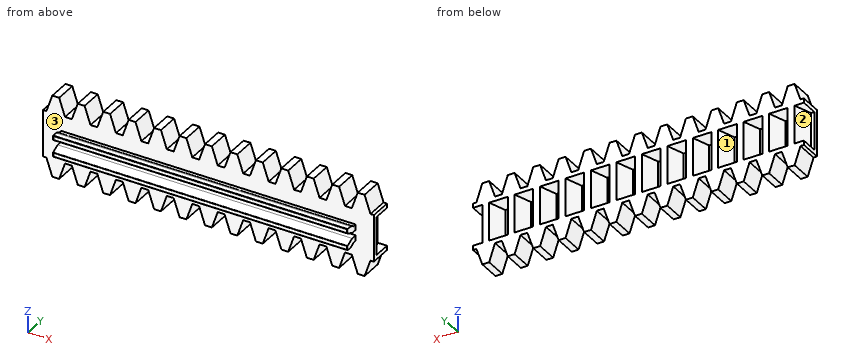
```python
from build123d import *

# Parameters (mm, degrees)
SKETCH_1_W                     = 4.65
SKETCH_1_H                     = 8.6
EXTRUDE_1_DEPTH                = 4
EXTRUDE_2_DEPTH                = 4
CUT_EXTRUDE_1_DEPTH            = 3.5
PATTERN_LINEAR_4_COUNT         = 13
PATTERN_LINEAR_4_PITCH         = 4.65
PATTERN_LINEAR_4_COPY_1_DEPTH  = 4
PATTERN_LINEAR_4_COPY_2_DEPTH  = 4
PATTERN_LINEAR_4_COPY_3_DEPTH  = 4
PATTERN_LINEAR_4_COPY_4_DEPTH  = 4
PATTERN_LINEAR_4_COPY_5_DEPTH  = 4
PATTERN_LINEAR_4_COPY_6_DEPTH  = 4
PATTERN_LINEAR_4_COPY_7_DEPTH  = 4
PATTERN_LINEAR_4_COPY_8_DEPTH  = 4
PATTERN_LINEAR_4_COPY_9_DEPTH  = 4
PATTERN_LINEAR_4_COPY_10_DEPTH = 4
PATTERN_LINEAR_4_COPY_11_DEPTH = 4
PATTERN_LINEAR_4_COPY_12_DEPTH = 4
EXTRUDE_START                  = 1
EXTRUDE_4_DEPTH                = 53.8
FILLET_1_R                     = 0.1


with BuildPart() as part:
    # 草图1 → 凸台-拉伸1 (new body)
    with BuildSketch(Plane(origin=(0, 0, 0), x_dir=(1, 0, 0), z_dir=(0, 1, 0))):
        Rectangle(SKETCH_1_W, SKETCH_1_H)
    extrude_1 = extrude(amount=EXTRUDE_1_DEPTH)

    # 草图3 → 凸台-拉伸2 (add)
    with BuildSketch(Plane(origin=(0, 0, 0), x_dir=(1, 0, 0), z_dir=(0, 1, 0))):
        Polygon((0.625, 7.5), (-0.625, 7.5), (-1.7, 4.3), (1.7, 4.3), align=None)
    extrude_2 = extrude(amount=EXTRUDE_2_DEPTH)

    # 镜向1: 凸台-拉伸2 across plane
    add(extrude_2.mirror(Plane.XY))

    # 草图4 → 切除-拉伸1 (cut, symmetric)
    with BuildSketch(Plane.XY):
        Polygon((-0.625, 4), (-2.325, 4), (-2.325, 0.8), (-1.7, 0.8), align=None)
        Polygon((1.7, 0.8), (2.325, 0.8), (2.325, 4), (0.625, 4), align=None)
    cut_extrude_1 = extrude(amount=CUT_EXTRUDE_1_DEPTH, both=True, mode=Mode.SUBTRACT)

    # 阵列(线性)4: 凸台-拉伸1, 凸台-拉伸2, 切除-拉伸1 ×13
    with Locations(*[(i * PATTERN_LINEAR_4_PITCH, 0, 0) for i in range(1, PATTERN_LINEAR_4_COUNT)]):
        add(extrude_1)
        add(extrude_2)
        add(cut_extrude_1, mode=Mode.SUBTRACT)

    # 阵列(线性)4 copy 1 sketch → 阵列(线性)4 copy 1 (add)
    with BuildSketch(Plane(origin=(4.65, 0, 0), x_dir=(1, 0, 0), z_dir=(0, 1, 0))):
        Polygon((0.625, -7.5), (-0.625, -7.5), (-1.7, -4.3), (1.7, -4.3), align=None)
    extrude(amount=PATTERN_LINEAR_4_COPY_1_DEPTH)

    # 阵列(线性)4 copy 2 sketch → 阵列(线性)4 copy 2 (add)
    with BuildSketch(Plane(origin=(9.3, 0, 0), x_dir=(1, 0, 0), z_dir=(0, 1, 0))):
        Polygon((0.625, -7.5), (-0.625, -7.5), (-1.7, -4.3), (1.7, -4.3), align=None)
    extrude(amount=PATTERN_LINEAR_4_COPY_2_DEPTH)

    # 阵列(线性)4 copy 3 sketch → 阵列(线性)4 copy 3 (add)
    with BuildSketch(Plane(origin=(13.95, 0, 0), x_dir=(1, 0, 0), z_dir=(0, 1, 0))):
        Polygon((0.625, -7.5), (-0.625, -7.5), (-1.7, -4.3), (1.7, -4.3), align=None)
    extrude(amount=PATTERN_LINEAR_4_COPY_3_DEPTH)

    # 阵列(线性)4 copy 4 sketch → 阵列(线性)4 copy 4 (add)
    with BuildSketch(Plane(origin=(18.6, 0, 0), x_dir=(1, 0, 0), z_dir=(0, 1, 0))):
        Polygon((0.625, -7.5), (-0.625, -7.5), (-1.7, -4.3), (1.7, -4.3), align=None)
    extrude(amount=PATTERN_LINEAR_4_COPY_4_DEPTH)

    # 阵列(线性)4 copy 5 sketch → 阵列(线性)4 copy 5 (add)
    with BuildSketch(Plane(origin=(23.25, 0, 0), x_dir=(1, 0, 0), z_dir=(0, 1, 0))):
        Polygon((0.625, -7.5), (-0.625, -7.5), (-1.7, -4.3), (1.7, -4.3), align=None)
    extrude(amount=PATTERN_LINEAR_4_COPY_5_DEPTH)

    # 阵列(线性)4 copy 6 sketch → 阵列(线性)4 copy 6 (add)
    with BuildSketch(Plane(origin=(27.9, 0, 0), x_dir=(1, 0, 0), z_dir=(0, 1, 0))):
        Polygon((0.625, -7.5), (-0.625, -7.5), (-1.7, -4.3), (1.7, -4.3), align=None)
    extrude(amount=PATTERN_LINEAR_4_COPY_6_DEPTH)

    # 阵列(线性)4 copy 7 sketch → 阵列(线性)4 copy 7 (add)
    with BuildSketch(Plane(origin=(32.55, 0, 0), x_dir=(1, 0, 0), z_dir=(0, 1, 0))):
        Polygon((0.625, -7.5), (-0.625, -7.5), (-1.7, -4.3), (1.7, -4.3), align=None)
    extrude(amount=PATTERN_LINEAR_4_COPY_7_DEPTH)

    # 阵列(线性)4 copy 8 sketch → 阵列(线性)4 copy 8 (add)
    with BuildSketch(Plane(origin=(37.2, 0, 0), x_dir=(1, 0, 0), z_dir=(0, 1, 0))):
        Polygon((0.625, -7.5), (-0.625, -7.5), (-1.7, -4.3), (1.7, -4.3), align=None)
    extrude(amount=PATTERN_LINEAR_4_COPY_8_DEPTH)

    # 阵列(线性)4 copy 9 sketch → 阵列(线性)4 copy 9 (add)
    with BuildSketch(Plane(origin=(41.85, 0, 0), x_dir=(1, 0, 0), z_dir=(0, 1, 0))):
        Polygon((0.625, -7.5), (-0.625, -7.5), (-1.7, -4.3), (1.7, -4.3), align=None)
    extrude(amount=PATTERN_LINEAR_4_COPY_9_DEPTH)

    # 阵列(线性)4 copy 10 sketch → 阵列(线性)4 copy 10 (add)
    with BuildSketch(Plane(origin=(46.5, 0, 0), x_dir=(1, 0, 0), z_dir=(0, 1, 0))):
        Polygon((0.625, -7.5), (-0.625, -7.5), (-1.7, -4.3), (1.7, -4.3), align=None)
    extrude(amount=PATTERN_LINEAR_4_COPY_10_DEPTH)

    # 阵列(线性)4 copy 11 sketch → 阵列(线性)4 copy 11 (add)
    with BuildSketch(Plane(origin=(51.15, 0, 0), x_dir=(1, 0, 0), z_dir=(0, 1, 0))):
        Polygon((0.625, -7.5), (-0.625, -7.5), (-1.7, -4.3), (1.7, -4.3), align=None)
    extrude(amount=PATTERN_LINEAR_4_COPY_11_DEPTH)

    # 阵列(线性)4 copy 12 sketch → 阵列(线性)4 copy 12 (add)
    with BuildSketch(Plane(origin=(55.8, 0, 0), x_dir=(1, 0, 0), z_dir=(0, 1, 0))):
        Polygon((0.625, -7.5), (-0.625, -7.5), (-1.7, -4.3), (1.7, -4.3), align=None)
    extrude(amount=PATTERN_LINEAR_4_COPY_12_DEPTH)

    # 草图6 → 凸台-拉伸4 (add)
    with BuildSketch(Plane(origin=(0, 0, 0), x_dir=(0, 0, -1), z_dir=(1, 0, 0)).offset(EXTRUDE_START)):
        with BuildLine():
            Line((1.5, 0), (0.5, 0))
            Line((0.5, 0), (0.5, -1.07225346))
            Line((0.5, -1.07225346), (1.165769145, -2.5))
            Line((1.165769145, -2.5), (1.95, -2.5))
            Line((1.95, -2.5), (1.95, -1.555590279))
            ThreePointArc((1.95, -1.555590279), (1.780042303, -1.088161527), (1.5, -0.677124344))
            Line((1.5, -0.677124344), (1.5, 0))
        make_face()
        with BuildLine():
            Line((-0.5, -1.07225346), (-1.165769145, -2.5))
            Line((-1.165769145, -2.5), (-1.95, -2.5))
            Line((-1.95, -2.5), (-1.95, -1.555590279))
            ThreePointArc((-1.95, -1.555590279), (-1.780042303, -1.088161527), (-1.5, -0.677124344))
            Line((-1.5, -0.677124344), (-1.5, 0))
            Line((-1.5, 0), (-0.5, 0))
            Line((-0.5, 0), (-0.5, -1.07225346))
        make_face()
    extrude(amount=EXTRUDE_4_DEPTH)

    # 圆角1
    fillet_1_edges = [part.edges().sort_by_distance(p)[0] for p in [
        (1, -2.5, -1.557884573),
        (27.9, -2.5, -1.165769145),
        (27.9, -2.5, -1.95),
        (54.8, -2.5, -1.557884573),
        (1, -2.5, 1.557884573),
        (27.9, -2.5, 1.95),
        (27.9, -2.5, 1.165769145),
        (54.8, -2.5, 1.557884573),
    ]]
    fillet(fillet_1_edges, radius=FILLET_1_R)


solid = part.part
```
The listing builds one solid part. Answer for the finished solid, in the listing's coordinates (mm). Face numbers are marked on the shaded views. Round coordinates to 2 decimals unless told otherwise and drop trailing zeros. Loops run counter-clockwise (first coordinate to the right, second up) from the corner with the lowest first, then second, coordinate; pieces in that order, holes last.
Q1. Given pin 1 Ø0.6 at (x, y) = (49, 1.5) entering from -Z; pin 2 Ø0.6 at (x, z) = (35, -1.5) entering from +Y; pin 3 Ø2 at (x, z) = (43.5, -3.5) entering from -Y; pin 4 Ø2 at (y, z) = (-2, -4) entering from -X, each flat-ended and moving along its own axis, determine where each tip first touches the part or whether it passes through.
Q2. Section B-B, the plane z = 6.75 is taken. Count the separate pieces of the cut face and the enclosed holes in it, then the cut area to 3 significant figures.
Q3. Find the intervals of material crossed by line 1 (Z direction, x = 25, y = 1.75); line 2 (Z direction, x = 7.5, y = -0.25); line 3 (Y direction, x = 25, z = 3.25), in increasing order.
Q4. For a pull along X with two mould halves and no side action, classify the marked faces 1, 2 and 3 as released by +X, released by -X, zero draft, split by the parting line, or undercut.
Q5. Section A-A, the plane x = 14 is taken. Determine the outline of the cut face in (y, z).
Completed:
1. pin 1: stops at z = -4.3
1. pin 2: stops at y = 0.8
1. pin 3: stops at y = 0
1. pin 4: passes through
2. separate pieces: 13
2. enclosed holes: 0
2. area: 91.2 mm2
3. line 1: z = -4.3 to -3.5, 3.5 to 4.3
3. line 2: z = -1.5 to -0.5, 0.5 to 1.5
3. line 3: y = 0 to 0.8
4. face 1: undercut
4. face 2: released by -X
4. face 3: zero draft
5. outline: (-2.5, -1.85) arc R0.1 ccw to (-2.4, -1.95) - (-1.56, -1.95) arc R2 ccw to (-0.68, -1.5) - (0, -1.5) - (0, -7.5) - (4, -7.5) - (4, 7.5) - (0, 7.5) - (0, 1.5) - (-0.68, 1.5) arc R2 ccw to (-1.56, 1.95) - (-2.4, 1.95) arc R0.1 ccw to (-2.5, 1.85) - (-2.5, 1.23) arc R0.1 ccw to (-2.44, 1.14) - (-1.07, 0.5) - (0, 0.5) - (0, -0.5) - (-1.07, -0.5) - (-2.44, -1.14) arc R0.1 ccw to (-2.5, -1.23) - close
